Verification items for this drawing (mm, ordinates from the low corner). A direction names the side the tool comes from. Round coordinates to 2 decimals unless told otherwise and drop trailing zeros. Loops run counter-clockwise (first coordinate to the right, second up) from the corner with the lowest first, then second, coordinate; pieces in that order, holes last. Notation, with made-up numbers: (57.25, -22) - (78.25, -22) arc R9 ccw to (78.25, -12) - close; hole circle Ø3 at (-34.5, 56). An arc over 180 degrees is marked (long way). Put each result on its own line as item: value.
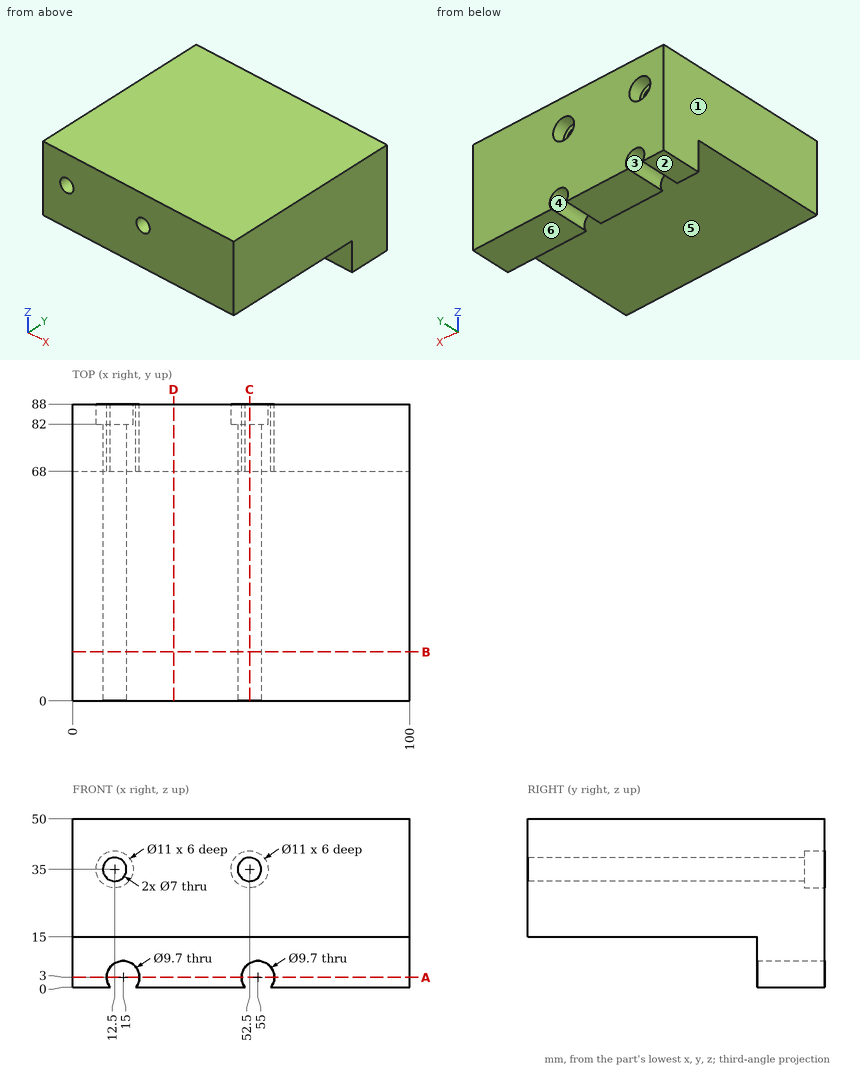
Item 1: Section check C-C on x = 52.5. Enter the section's corners in (y, z), then the cut area to 3 significant figures.
Filled sheet:
outline: (0, 15) - (68, 15) - (68, 7.16) - (88, 7.16) - (88, 29.5) - (82, 29.5) - (82, 31.5) - (0, 31.5) - close; (0, 38.5) - (82, 38.5) - (82, 40.5) - (88, 40.5) - (88, 50) - (0, 50) - close
area: 2,600 mm²
Item 2: Tool access check on the marked faces 5 and 6. Record the directions out of +Z, -Z, +X, -X, +Y, -Y that give a thin tool (end or side, any length) a straight path to the whole face; none if there is none.
Filled sheet:
face 5: -Z, +X, -X, -Y
face 6: -Z, +X, -X, +Y, -Y
Item 3: Go/stop test with flat-tipped pins: pin 1 (1 mm diameter, centred on x = 54, z = 31, fed in from +Y); pin 2 (1.5 mm diameter, centred on x = 47, y = 52, fed in from -Z); pin 3 (7.5 mm diameter, centred on x = 60.5, z = 10, fed in from -Y); pin 4 (5.5 mm diameter, centred on x = 52.5, z = 35, fed in from +Y). Record where each tip stops, or that it passes through.
Filled sheet:
pin 1: y = 82
pin 2: z = 15
pin 3: y = 68
pin 4: through
Item 4: Section check D-D on x = 30. Enter the section's corners in (y, z), then the cut area to 3 significant figures.
Filled sheet:
outline: (0, 15) - (68, 15) - (68, 0) - (88, 0) - (88, 50) - (0, 50) - close
area: 3,380 mm²
Item 5: Section check A-A on z = 3. Enter the section's corners in (x, y).
Filled sheet:
outline: (0, 68) - (10.15, 68) - (10.15, 88) - (0, 88) - close; (19.85, 68) - (50.15, 68) - (50.15, 88) - (19.85, 88) - close; (59.85, 68) - (100, 68) - (100, 88) - (59.85, 88) - close
Item 6: Thickness scan on line 1 (X direction, y = 22, z = 34); line 2 (Z direction, x = 52.5, y = 35.5); line 3 (X direction, y = 77.5, z = 5). Record the ranges inside material, lowest first. Write a range as from..to.
Filled sheet:
line 1: 0..9.15, 15.85..49.15, 55.85..100
line 2: 15..31.5, 38.5..50
line 3: 0..10.58, 19.42..50.58, 59.42..100
Item 7: Release check for a two-part mould opening along X. For the marked faces 1, 2, 3 and 4 record: +X half, -X half, draft (parallel to the pull), parting line (faces both ways), or undercut.
Filled sheet:
face 1: -X half
face 2: draft
face 3: undercut
face 4: undercut
Item 8: Section check B-B on y = 14.5. Enter the section's corners in (x, z), then the cut area to 3 significant figures.
Filled sheet:
outline: (0, 15) - (100, 15) - (100, 50) - (0, 50) - close; hole circle Ø7 at (12.5, 35); hole circle Ø7 at (52.5, 35)
area: 3,420 mm²
